Part model, mm, in its own coordinate system. Round coordinates to 2 decimals unless told otherwise and drop trailing zeros. Loops run counter-clockwise (first coordinate to the right, second up) from the corner with the lowest first, then second, coordinate; pieces in that order, holes last. Notation, with made-up numbers: (-38.75, 74) -> (1.25, 74) arc R23 ccw to (1.25, 90) -> close; hole circle Ø4 at (59, 31.5). An arc over 180 degrees is marked (long way). Use a Markdown table: item, result. Add a question column.
Item 1: Cut at C-C, the plane z = 2.75. List the corners of the cut face in (x, y).
Item 2: Two-plate mould, pull along X, no slides. Class faces 1 (the face through (-39.7, 1, 3)), 2 (the face through (1, 18, 6.35)), 3 (the face through (39.7, -1, 3)), 4 (the face through (-0.28, -21.68, 3.13)): pulls with the +X half, pulls with the -X half, needs draft (parallel to the pull), parting line crosses it, or undercut.
Item 3: Cut at B-B, the plane y = 0. List the corners of the cut face in (x, z), plus the area to 3 significant figures.
Item 4: Probe line 1 (Y direction, x = 20, z = 1); line 2 (X direction, y = 1, z = 0.5) (3 decimals); line 3 (Y direction, x = -7, z = 4.25). List the from-to ranges inside material, lowest first. Write a range as [from, to].
Item 5: Cut at D-D, the plane x = -20. List the corners of the cut face in (y, z), plus the area to 3 significant figures.
Item 6: Cut at A-A, the plane x = 0. List the corners of the cut face in (y, z).
```python
from build123d import *

# Parameters (mm, degrees)
BOSS_EXTRUDE1_DEPTH = 6.35


with BuildPart() as part:
    # Sketch1 → Boss-Extrude1 (new body)
    with BuildSketch(Plane.XY):
        Polygon((0, 39.0525), (39.7, 39.0525), (39.7, 0), (39.7, -39.0525), (0, -39.0525), (-39.7, -39.0525), (-39.7, 0), (-39.7, 39.0525), align=None)
        with BuildLine():
            ThreePointArc((2.15265, 23.8125), (0, 25.96515), (-2.15265, 23.8125))
            ThreePointArc((-2.15265, 23.8125), (0, 21.65985), (2.15265, 23.8125))
        make_face(mode=Mode.SUBTRACT)
        with BuildLine():
            ThreePointArc((-14.3, 0), (0, -14.3), (14.3, 0))
            ThreePointArc((14.3, 0), (0, 14.3), (-14.3, 0))
        make_face(mode=Mode.SUBTRACT)
        with BuildLine():
            ThreePointArc((-22.774879928, 11.90625), (-20.622229928, 9.7536), (-18.469579928, 11.90625))
            ThreePointArc((-18.469579928, 11.90625), (-20.622229928, 14.0589), (-22.774879928, 11.90625))
        make_face(mode=Mode.SUBTRACT)
        with BuildLine():
            ThreePointArc((-22.774879928, -11.90625), (-20.622229928, -14.0589), (-18.469579928, -11.90625))
            ThreePointArc((-18.469579928, -11.90625), (-20.622229928, -9.7536), (-22.774879928, -11.90625))
        make_face(mode=Mode.SUBTRACT)
        with BuildLine():
            ThreePointArc((-2.15265, -23.8125), (0, -25.96515), (2.15265, -23.8125))
            ThreePointArc((2.15265, -23.8125), (0, -21.65985), (-2.15265, -23.8125))
        make_face(mode=Mode.SUBTRACT)
        with BuildLine():
            ThreePointArc((18.469579928, 11.90625), (20.622229928, 9.7536), (22.774879928, 11.90625))
            ThreePointArc((22.774879928, 11.90625), (20.622229928, 14.0589), (18.469579928, 11.90625))
        make_face(mode=Mode.SUBTRACT)
        with BuildLine():
            ThreePointArc((18.469579928, -11.90625), (20.622229928, -14.0589), (22.774879928, -11.90625))
            ThreePointArc((22.774879928, -11.90625), (20.622229928, -9.7536), (18.469579928, -11.90625))
        make_face(mode=Mode.SUBTRACT)
    extrude(amount=BOSS_EXTRUDE1_DEPTH)


solid = part.part
```
A:
| question | item | result |
|---|---|---|
| 1 | outline | (-39.7, -39.05) -> (39.7, -39.05) -> (39.7, 39.05) -> (-39.7, 39.05) -> close; hole circle Ø4.31 at (-20.62, -11.91); hole circle Ø4.31 at (-20.62, 11.91); hole circle Ø28.6 at (0, 0); hole circle Ø4.31 at (0, -23.81); hole circle Ø4.31 at (0, 23.81); hole circle Ø4.31 at (20.62, -11.91); hole circle Ø4.31 at (20.62, 11.91) |
| 2 | face 1 | pulls with the -X half |
| 2 | face 2 | needs draft |
| 2 | face 3 | pulls with the +X half |
| 2 | face 4 | undercut |
| 3 | outline | (-39.7, 0) -> (-14.3, 0) -> (-14.3, 6.35) -> (-39.7, 6.35) -> close; (14.3, 0) -> (39.7, 0) -> (39.7, 6.35) -> (14.3, 6.35) -> close |
| 3 | area | 323 mm^2 |
| 4 | line 1 | y = [-39.05, -13.97], [-9.85, 9.85], [13.97, 39.05] |
| 4 | line 2 | x = [-39.7, -14.265], [14.265, 39.7] |
| 4 | line 3 | y = [-39.05, -12.47], [12.47, 39.05] |
| 5 | outline | (-39.05, 0) -> (-13.97, 0) -> (-13.97, 6.35) -> (-39.05, 6.35) -> close; (-9.85, 0) -> (9.85, 0) -> (9.85, 6.35) -> (-9.85, 6.35) -> close; (13.97, 0) -> (39.05, 0) -> (39.05, 6.35) -> (13.97, 6.35) -> close |
| 5 | area | 444 mm^2 |
| 6 | outline | (-39.05, 0) -> (-25.97, 0) -> (-25.97, 6.35) -> (-39.05, 6.35) -> close; (-21.66, 0) -> (-14.3, 0) -> (-14.3, 6.35) -> (-21.66, 6.35) -> close; (14.3, 0) -> (21.66, 0) -> (21.66, 6.35) -> (14.3, 6.35) -> close; (25.97, 0) -> (39.05, 0) -> (39.05, 6.35) -> (25.97, 6.35) -> close |
